```python
from build123d import *

# Parameters (mm, degrees)
EXTRUDE_1_DEPTH          = 23
SKETCH_2_R               = 2.5
CUT_EXTRUDE_1_DEPTH      = 4
CUT_EXTRUDE_1_DEPTH_BACK = 6.175426481
HOLE_WIZARD_M41_D        = 4.5
CHAMFER_1_SIZE           = 1
CHAMFER_1_SIZE2          = 2


with BuildPart() as part:
    # Эскиз1 → Бобышка-Вытянуть1 (new body)
    with BuildSketch(Plane.XY):
        Polygon((0, 0), (-12.29, 0), (-12.29, 1.5), (-11.574573519, 1.5), (-11.574573519, 10.5), (-13.574573519, 10.5), (-16.75, 16), (0, 16), align=None)
    extrude(amount=EXTRUDE_1_DEPTH)

    # Эскиз2 → Вырез-Вытянуть1 (cut, two sides)
    with BuildSketch(Plane(origin=(-11.574573519, 0, 0), x_dir=(0, 0, -1), z_dir=(1, 0, 0))) as cut_extrude_1_sk:
        with Locations((-19, 5)):
            Circle(SKETCH_2_R)
        with Locations((-4, 5)):
            Circle(SKETCH_2_R)
    extrude(amount=CUT_EXTRUDE_1_DEPTH, mode=Mode.SUBTRACT)
    extrude(cut_extrude_1_sk.sketch, amount=-CUT_EXTRUDE_1_DEPTH_BACK, mode=Mode.SUBTRACT)

    # Отверстие с зазором M41 (through all)
    with Locations(Plane(origin=(0, 1.542761086, 4.525415006), x_dir=(0, 0, 1), z_dir=(1, 0, 0))):
        with Locations((6.974584994, -3.457238914)):
            Hole(HOLE_WIZARD_M41_D / 2)

    # Фаска1
    chamfer_1_edges = [part.edges().sort_by_distance(p)[0] for p in [
        (-16.75, 16, 11.5),
    ]]
    chamfer_1_side = [part.faces().sort_by_distance(p)[0] for p in [
        (-8.375, 16, 11.5),
    ]]
    chamfer(chamfer_1_edges, length=CHAMFER_1_SIZE, length2=CHAMFER_1_SIZE2, reference=chamfer_1_side[0])


solid = part.part
```
Work out the finished part from the listing and answer in its coordinate system (mm). A direction names the side the tool comes from. Coordinates: 2 decimals unless noted, no trailing zeros. Write each loop counter-clockwise with the first axis right and the second up, starting at its lowest first coordinate (ties: lowest second). Pieces come first, ordered by that corner, then holes. Notation, with made-up numbers: (-10.75, 63) - (34.25, 63) arc R30 ccw to (34.25, 102) - close; hole circle Ø11 at (82, 66.25). An arc over 180 degrees is marked (long way). Answer as a JSON object with one key per item and string values.
Q1. Find section A-A (z = 11.5). Write down the section's boundary in (x, y).
Results list:
{"outline": "(-15.75, 14.27) - (-13.57, 10.5) - (-11.57, 10.5) - (-11.57, 7.25) - (0, 7.25) - (0, 16) - (-15.75, 16) - close; (-12.29, 0) - (0, 0) - (0, 2.75) - (-11.57, 2.75) - (-11.57, 1.5) - (-12.29, 1.5) - close"}
Q2. Find section C-C (x = -11). Write down the section's boundary in (y, z), plus the area to 3 significant figures.
Results list:
{"outline": "(0, 0) - (16, 0) - (16, 23) - (0, 23) - close; hole circle Ø5 at (5, 4); hole circle Ø5 at (5, 19); hole circle Ø4.5 at (5, 11.5)", "area": "313 mm^2"}
Q3. Find section B-B (y = 5). Write down the section's boundary in (x, z).
Results list:
{"outline": "(-11.57, 0) - (0, 0) - (0, 9.25) - (-11.57, 9.25) - (-11.57, 6.5) - (-7.57, 6.5) - (-7.57, 1.5) - (-11.57, 1.5) - close; (-11.57, 13.75) - (0, 13.75) - (0, 23) - (-11.57, 23) - (-11.57, 21.5) - (-7.57, 21.5) - (-7.57, 16.5) - (-11.57, 16.5) - close"}
Q4. For a pull along Y with two mould halves and no side action, classify faces 1 (the cylindrical face through (-9.603, 5.751, 1.615)), 2 (the flat face through (-6, 8, 0)), 3 (the flat face through (-8, 16, 11)), 4 (the flat face through (-7.575, 5, 4)) as pulls with the +Y half, pulls with the -Y half, needs draft (parallel to the pull), parting line crosses it, or undercut.
Results list:
{"face 1": "undercut", "face 2": "needs draft", "face 3": "pulls with the +Y half", "face 4": "undercut"}
Q5. Which of the six approach directions +Z, -Z, +X, -X, +Y, -Y give full straight-line access (tool end or side, diameter ignored) to faces 5 (the flat face through (-12.29, 1, 11)), 6 (the flat face through (-6, 0, 11)), 7 (the flat face through (0, 8, 11)), 8 (the flat face through (-11.575, 8, 11)), 9 (the flat face through (-7.575, 5, 19))?
Results list:
{"face 5": "+Z, -Z, -X, -Y", "face 6": "+Z, -Z, +X, -X, -Y", "face 7": "+Z, -Z, +X, +Y, -Y", "face 8": "+Z, -Z, -X", "face 9": "-X"}
Q6. Find section D-D (x = -0.75). Write down the section's boundary in (y, z).
Results list:
{"outline": "(0, 0) - (16, 0) - (16, 23) - (0, 23) - close; hole circle Ø4.5 at (5, 11.5)"}
Q7. Given pin 1 Ø4 at (y, z) = (5, 18) entering from -X; pin 2 Ø1.2 at (y, z) = (0.5, 8.5) entering from -X; pin 3 Ø4 at (y, z) = (5, 4) entering from -X, each flat-ended and moving along its own axis, determine where each tip first touches the part or whether it passes through.
Results list:
{"pin 1": "stops at x = -11.57", "pin 2": "stops at x = -12.29", "pin 3": "stops at x = -7.57"}
Q8. Consider L1, parallel to Y at x = -12, z = 5.75; L2, parallel to Y at x = -7, z = 11.5; L3, parallel to X at y = 9.5, z = 9.5. Determine where each line is inside the solid, lowest interval first. Write a range as from..to.
Results list:
{"L1": "y = 0..1.5, 10.5..16", "L2": "y = 0..2.75, 7.25..16", "L3": "x = -11.57..0"}
